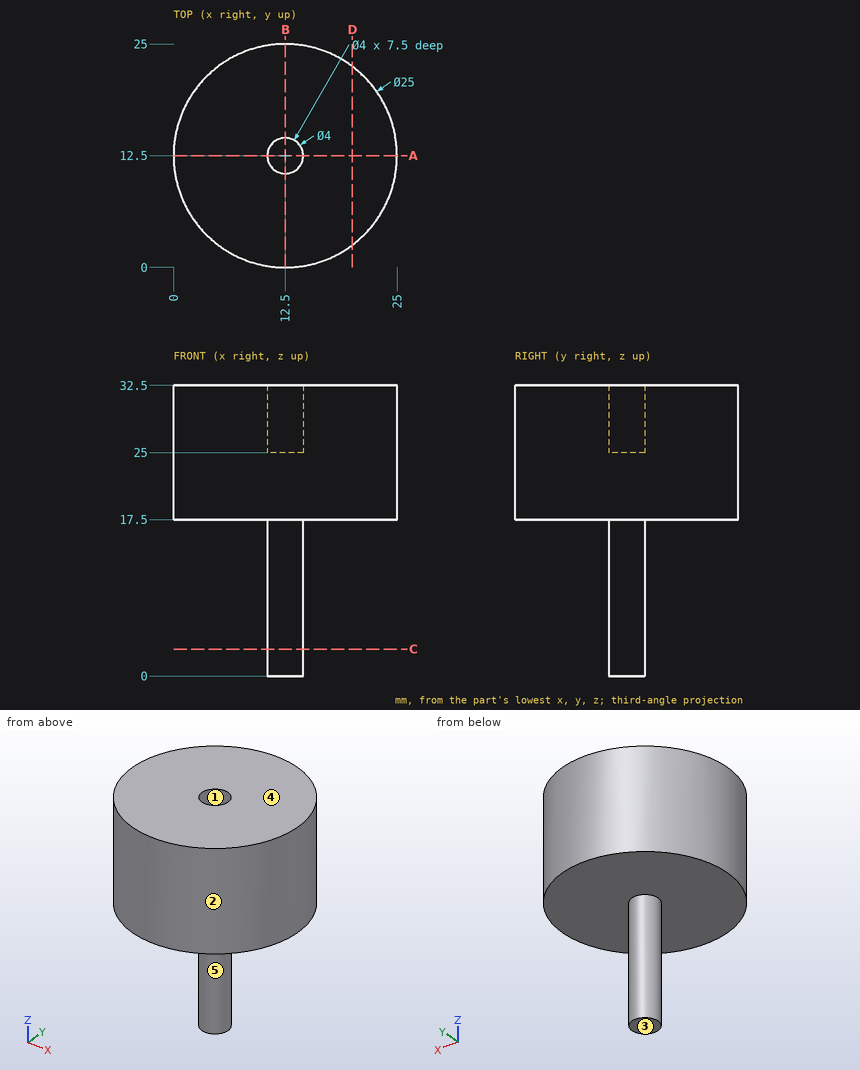
Source: three-view drawing plus pictorial views. Frame: mm from the lowest corner of the part. A direction names the side the tool comes from. Round coordinates to 2 decimals unless told otherwise and drop trailing zeros. Loops run counter-clockwise (first coordinate to the right, second up) from the corner with the lowest first, then second, coordinate; pieces in that order, holes last.
1. Section query A-A on y = 12.5. Output: boundary loops of the cut face in (x, z), and give its area (3 significant figures).
2. Contact query for flat-ended pins moving along their axis: pin 1 (3 mm diameter, centred on x = 10.5, z = 8, fed in from +Y); pin 2 (8 mm diameter, centred on x = 7, y = 22, fed in from -Z); pin 3 (1.5 mm diameter, centred on x = 8, z = 28.5, fed in from +Y). Output: stop coordinate, or through.
3. Mould query, pull axis Y, two halves, no side actions, for the marked faces 1, 2 and 3. Classes: released by +Y, released by -Y, zero draft, split by the parting line, or undercut.
4. Section query C-C on z = 3. Output: boundary loops of the cut face in (x, y).
5. Section query D-D on x = 20. Output: boundary loops of the cut face in (y, z).
6. Ray query, L1, parallel to Y at x = 12.5, z = 28.5; L2, parallel to Z at x = 3, y = 18.5; L3, parallel to Y at x = 14, z = 30. Return the intervals inside material, ascending.
7. Access query for the marked faces 4 and 5. Directions: +Z, -Z, +X, -X, +Y, -Y. A direction counts if a zero-diameter tool reaches every point of the face in a straight line with its end or side. Return the directions, or none.
Answers below:
1. outline: (0, 17.5) - (10.5, 17.5) - (10.5, 0) - (14.5, 0) - (14.5, 17.5) - (25, 17.5) - (25, 32.5) - (14.5, 32.5) - (14.5, 25) - (10.5, 25) - (10.5, 32.5) - (0, 32.5) - close
1. area: 415 mm2
2. pin 1: stops at y = 14.44
2. pin 2: stops at z = 17.5
2. pin 3: stops at y = 24.42
3. face 1: undercut
3. face 2: split by the parting line
3. face 3: zero draft
4. outline: circle Ø4 at (12.5, 12.5)
5. outline: (2.5, 17.5) - (22.5, 17.5) - (22.5, 32.5) - (2.5, 32.5) - close
6. L1: y = 0 to 10.5, 14.5 to 25
6. L2: z = 17.5 to 32.5
6. L3: y = 0.09 to 11.18, 13.82 to 24.91
7. face 4: +Z, +X, -X, +Y, -Y
7. face 5: -Z
